from build123d import *

# Parameters (mm, degrees)
SKETCH1_R                = 110
BOSS_EXTRUDE1_DEPTH      = 22
BOSS_EXTRUDE2_DEPTH      = 120
BOSS_EXTRUDE2_DEPTH_BACK = 22
SKETCH2_R                = 60
CUT_EXTRUDE3_DEPTH       = 211.627633515
CUT_EXTRUDE3_DEPTH_BACK  = 120
SKETCH3_R                = 50
FILLET1_R                = 3


with BuildPart() as part:
    # Sketch1 → Boss-Extrude1 (new body)
    with BuildSketch(Plane.XY):
        Circle(SKETCH1_R)
    extrude(amount=BOSS_EXTRUDE1_DEPTH)

    # Sketch2 → Boss-Extrude2 (add, two sides: drawn at the far end of the back side and taken through both)
    with BuildSketch(Plane.XY.offset(22).offset(-BOSS_EXTRUDE2_DEPTH_BACK)):
        Circle(SKETCH2_R)
    extrude(amount=BOSS_EXTRUDE2_DEPTH + BOSS_EXTRUDE2_DEPTH_BACK)

    # Sketch3 → Cut-Extrude3 (cut, two sides: drawn at the far end of the back side and taken through both)
    with BuildSketch(Plane.XY.offset(-CUT_EXTRUDE3_DEPTH_BACK)):
        Circle(SKETCH3_R)
    extrude(amount=CUT_EXTRUDE3_DEPTH + CUT_EXTRUDE3_DEPTH_BACK, mode=Mode.SUBTRACT)

    # Fillet1
    fillet1_edges = [part.edges().sort_by_distance(p)[0] for p in [
        (-60, 0, 22),
    ]]
    fillet(fillet1_edges, radius=FILLET1_R)


solid = part.part
Could you check a few things on this model? Use its own coordinates, in mm. A direction names the side the tool comes from. Give positions to 0.01 mm unless a question says otherwise; leave off trailing zeros. Write each loop counter-clockwise with the first axis right and the second up, starting at its lowest first coordinate (ties: lowest second). Pieces come first, ordered by that corner, then holes. Notation, with made-up numbers: (-30, 4.25) -> (12, 4.25) arc R18 ccw to (12, 19.25) -> close; hole circle Ø8 at (6.25, 59). An arc over 180 degrees is marked (long way). Write each question's results on one line, items separated by ' | '. Start each with the question number.
Q1. Suppose I cut it at C-C, the plane z = 128. List the corners of the cut face in (x, y) for me.
Q2. I'm going to push flat-ended pins straight in: pin 1 Ø4 at (x, z) = (2, 46) entering from +Y; pin 2 Ø6 at (x, z) = (-19.5, 80) entering from +Y; pin 3 Ø6 at (y, z) = (52, 104) entering from -X. Where does each tip first touch, or does it pass through?
Q3. Which directions (+Z, -Z, +X, -X, +Y, -Y) give clear straight access to the entire face, cutting with the end or side of a thin tool? Please do faces 4 (the face through (23, -47, 0)), 5 (the face through (-59.94, 2.64, 82.68)).
Q4. Suppose I cut it at D-D, the plane y = 69. List the corners of the cut face in (x, z) for me, and give its area (3 significant figures).
Q5. Suppose I cut it at A-A, the plane x = 0. List the corners of the cut face in (y, z) for me, and give its area (3 significant figures).
Q6. I need wall thicknesses on probe 1 along X at (y, z) = (0, 85); probe 2 along Z at (x, y) = (19, -96.5). Which ranges of each line are inside material? Lowest first, please.
Q7. We'd pull the mould along X, two halves only. Please class faces 1 (the face through (-23.846, -107.384, 10.846)), 2 (the face through (-23, 45, 142)), 3 (the face through (47.69, 15.02, 70.01)): +X half, -X half, draft (parallel to the pull), parting line (faces both ways), or undercut.
Outcome:
1) outline: circle Ø120 at (0, 0); hole circle Ø100 at (0, 0)
2) pin 1: y = 60 | pin 2: y = 57.69 | pin 3: x = -34.63
3) face 4: -Z, +X, -X, +Y, -Y | face 5: +Z
4) outline: (-85.67, 0) -> (85.67, 0) -> (85.67, 22) -> (-85.67, 22) -> close | area: 3,770 mm2
5) outline: (-110, 0) -> (-50, 0) -> (-50, 142) -> (-60, 142) -> (-60, 25) arc R3 cw to (-63, 22) -> (-110, 22) -> close; (50, 0) -> (110, 0) -> (110, 22) -> (63, 22) arc R3 cw to (60, 25) -> (60, 142) -> (50, 142) -> close | area: 5,040 mm2
6) probe 1: -60 to -50, 50 to 60 | probe 2: 0 to 22
7) face 1: parting line | face 2: draft | face 3: undercut
